Verification items for the finished model (mm, model axes). Round coordinates to 2 decimals unless told otherwise and drop trailing zeros. Order: outer loops, then holes, each group sorted by start corner. A loop starts at its lowest first (then second) coordinate and runs counter-clockwise, first axis right, second up. Notation, with made-up numbers: (15.5, 73) -> (19.5, 73) arc R35 ccw to (19.5, 107) -> close; hole circle Ø7 at (57.5, 30). An arc over 180 degrees is marked (long way). Return JSON: item names as keys, results as strings. Group by question number.
Item 1: Sectioned sample at D-D on y = 41.5. Record the cut outline in (x, z), plus the area to 3 significant figures.
Item 2: Sectioned sample at C-C on y = -25.4. Record the cut outline in (x, z).
Item 3: Sectioned sample at B-B on z = 1.75. Record the cut outline in (x, y) (3 decimals), plus the area to 3 significant figures.
Item 4: Draft check along Y on faces 1 (the cylindrical face through (-9.42, -22.05, 1.29)), 2 (the cylindrical face through (38.971, -74.926, 1.252)), 3 (the flat face through (-1, 1, 2.54)). Enter one of: pulls with the +Y half, pulls with the -Y half, needs draft (parallel to the pull), parting line crosses it, or undercut.
Item 5: Depth check by flat-ended pin: pin 1 Ø8 at (x, y) = (-13.5, -23) entering from -Z. Enter the tip coordinate at first touch or a pass-through.
Item 6: Sectioned sample at A-A on x = -9.5. Record the cut outline in (y, z).
Item 7: Scan lines: probe 1 along Y at (x, z) = (-10.16, 0.95); probe 2 along Y at (x, z) = (-10, 1.85); probe 3 along X at (y, z) = (1, 1). Record each from-to range of solid material in increasing order. Write a range as from..to.
```python
from build123d import *

# Parameters (mm, degrees)
SKETCH1_R           = 84.455
BOSS_EXTRUDE1_DEPTH = 2.54
SKETCH2_R           = 3.429
CUT_EXTRUDE1_DEPTH  = 2.54


with BuildPart() as part:
    # Sketch1 → Boss-Extrude1 (new body)
    with BuildSketch(Plane.XY):
        Circle(SKETCH1_R)
    extrude(amount=BOSS_EXTRUDE1_DEPTH)

    # Sketch2 → Cut-Extrude1 (cut)
    with BuildSketch(Plane.XY.offset(2.54)):
        with Locations((-10.16, 25.4)):
            Circle(SKETCH2_R)
        with Locations(Location((10.16, 25.4, 0), (0, 0, 180))):
            Circle(SKETCH2_R)
        with Locations((10.16, -25.4)):
            Circle(SKETCH2_R)
        with Locations(Location((-10.16, -25.4, 0), (0, 0, 180))):
            Circle(SKETCH2_R)
    extrude(amount=-CUT_EXTRUDE1_DEPTH, mode=Mode.SUBTRACT)


solid = part.part
```
Recorded:
{
 "1": {"outline": "(-73.56, 0) -> (73.56, 0) -> (73.56, 2.54) -> (-73.56, 2.54) -> close", "area": "374 mm²"},
 "2": {"outline": "(-80.54, 0) -> (-13.59, 0) -> (-13.59, 2.54) -> (-80.54, 2.54) -> close; (-6.73, 0) -> (6.73, 0) -> (6.73, 2.54) -> (-6.73, 2.54) -> close; (13.59, 0) -> (80.54, 0) -> (80.54, 2.54) -> (13.59, 2.54) -> close"},
 "3": {"outline": "circle Ø168.91 at (0, 0); hole circle Ø6.858 at (-10.16, -25.4); hole circle Ø6.858 at (-10.16, 25.4); hole circle Ø6.858 at (10.16, -25.4); hole circle Ø6.858 at (10.16, 25.4)", "area": "22,300 mm²"},
 "4": {"face 1": "undercut", "face 2": "parting line crosses it", "face 3": "needs draft"},
 "5": {"pin 1": "z = 0"},
 "6": {"outline": "(-83.92, 0) -> (-28.76, 0) -> (-28.76, 2.54) -> (-83.92, 2.54) -> close; (-22.04, 0) -> (22.04, 0) -> (22.04, 2.54) -> (-22.04, 2.54) -> close; (28.76, 0) -> (83.92, 0) -> (83.92, 2.54) -> (28.76, 2.54) -> close"},
 "7": {"probe 1": "-83.84..-28.83, -21.97..21.97, 28.83..83.84", "probe 2": "-83.86..-28.83, -21.97..21.97, 28.83..83.86", "probe 3": "-84.45..84.45"}
}
